Design review of the part built by this model. Coordinates are the model's own, in mm. A direction names the side the tool comes from. Coordinates: 2 decimals unless noted, no trailing zeros. Loops run counter-clockwise (first coordinate to the right, second up) from the corner with the lowest first, then second, coordinate; pieces in that order, holes last. Notation, with made-up numbers: (10.25, -16) - (65.25, -16) arc R34 ccw to (65.25, 21) - close; hole circle Ø1 at (-11, 46). An arc over 180 degrees is marked (long way). Return JSON: item names as keys, results as strings. Group by question number.
Autodesk Inventor part; units mm, degrees
ref_plane "YZ Plane" through (0, 0, 0) normal (1, 0, 0) x (0, 1, 0)
ref_plane "XZ Plane" through (0, 0, 0) normal (0, 1, 0) x (-1, 0, 0)
ref_plane "XY Plane" through (0, 0, 0) normal (0, 0, 1) x (1, 0, 0)
sketch "Szkic1" plane through (0, 0, 0) normal (1, 0, 0) x (0, 1, 0)
  circle A0 centre (0, 0) radius 12.5
  dimension "d0" = 25
extrude "Wyciągnięcie proste1" add sketch "Szkic1" along normal blind 30
sketch "Szkic2" plane through (0, 0, 0) normal (-1, 0, 0) x (0, 0, 1)
  circle A0 centre (0, 0) radius 1.55
  dimension "d3" = 3.1
extrude "Wyciągnięcie proste2" cut sketch "Szkic2" against normal blind 30
sketch "Szkic4" plane through (0, 0, 0) normal (-1, 0, 0) x (0, 0, 1)
  circle A0 centre (0, 0) radius 12.5
  circle A1 centre (0, 0) radius 8.5
  dimension "d6" = 4
extrude "Wyciągnięcie proste3" cut sketch "Szkic4" against normal blind 15 contours A1
sketch "Szkic5" plane through (15, 0, 0) normal (-1, 0, 0) x (0, 0, 1)
  circle A0 centre (0, 0) radius 1.55
  circle A1 centre (0, 0) radius 1.55
  line L0 (-1.0392, -1.15) -> (1.0392, -1.15)
  point P0 (0, -1.15)
  point P1 (1.0392, -1.15)
  point P2 (-1.0392, -1.15)
  dimension "d9" = 1.15
extrude "Wyciągnięcie proste4" add sketch "Szkic5" against normal up to surface (15 mm away) contours L0 A0 picked at (-0.2431, -1.2226)
properties part number "kolo"
Item 1: Add section B-B (z = -7.5). State the section outline as (x, y) points.
Item 2: For faces 4 (the face through (0, -3, -8.2)), 5 (the face through (22, -1.15, 0)), 6 (the face through (7.395, 7.167, 4.57)), list the 3-axis set-ups (+Z, -Z, +X, -X, +Y, -Y) from which the entire face can be reached by the end or side of a thin tool; tool diameter is ignored.
Item 3: For P1, Ø12, axis at x = 4.5, z = -4.5, coming from the +Y side; P2, Ø3, axis at y = 4, z = -3.5, coming from the -X side; P3, Ø5, axis at x = 19.5, y = 8, coming from the -Z side (3 decimals); P4, Ø1.5, axis at x = 22.5, z = -10, coming from the -Y side, all flat-tipped, find the tip position at first contact; note any pin that passes through.
Item 4: Draft analysis for pull direction Z (two halves, no side actions). For faces 1 (the face through (15, 0, 2)), 2 (the face through (30, 0, -3)), 3 (the face through (14.79, 11.923, -3.755)), state which applies: pulls with the +Z half, pulls with the -Z half, needs draft (parallel to the pull), parting line crosses it, or undercut.
Item 5: To check wall thickness, follow line 1 (Z direction, x = 22.75, y = 0); line 2 (X direction, y = 4.25, z = -4); line 3 (Y direction, x = 10, z = 4). State the ranges of each line that lie inside material, in increasing order. Write a range as from..to.
Item 6: Add section C-C (y = 4.75). State the section outline as (x, z) points.
Item 7: Add section D-D (x = 7.75). State the section outline as (y, z) points, then the cut area to 3 significant figures.
Item 8: Add section A-A (z = 0). State the section outline as (x, y) points.
Answers below:
{
 "1": {"outline": "(0, -10) - (30, -10) - (30, 10) - (0, 10) - (0, 4) - (15, 4) - (15, -4) - (0, -4) - close"},
 "2": {"face 4": "+Z, -Z, -X, +Y, -Y", "face 5": "+X, -X", "face 6": "-X"},
 "3": {"P1": "stops at y = 12.5", "P2": "stops at x = 15", "P3": "stops at z = -11.225", "P4": "stops at y = -8.41"},
 "4": {"face 1": "undercut", "face 2": "needs draft", "face 3": "parting line crosses it"},
 "5": {"line 1": "z = -12.5..-1.55, 1.55..12.5", "line 2": "x = 15..30", "line 3": "y = -11.84..-7.5, 7.5..11.84"},
 "6": {"outline": "(0, -11.56) - (30, -11.56) - (30, 11.56) - (0, 11.56) - (0, 7.05) - (15, 7.05) - (15, -7.05) - (0, -7.05) - close"},
 "7": {"outline": "circle Ø25 at (0, 0); hole circle Ø17 at (0, 0)", "area": "264 mm^2"},
 "8": {"outline": "(0, -12.5) - (30, -12.5) - (30, -1.15) - (15, -1.15) - (15, -8.5) - (0, -8.5) - close; (0, 8.5) - (15, 8.5) - (15, 1.55) - (30, 1.55) - (30, 12.5) - (0, 12.5) - close"}
}
